Work out the finished part from the listing and answer in its coordinate system (mm). Face numbers are marked on the shaded views. Round coordinates to 2 decimals unless told otherwise and drop trailing zeros. Order: outer loops, then holes, each group sorted by start corner. A loop starts at its lowest first (then second) coordinate and runs counter-clockwise, first axis right, second up. Notation, with made-up numbers: (11.5, 76) - (68.5, 76) arc R35 cw to (68.5, 110) - close; hole circle Ø2 at (45.25, -7.75). An arc over 180 degrees is marked (long way). Answer in a Markdown table with one row per item.
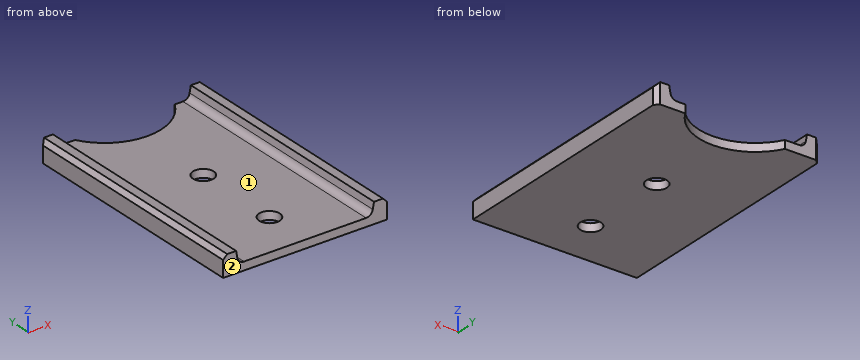
from build123d import *

# Parameters (mm, degrees)
F1_DEPTH = 228.6
F2_SIZE  = 3.81
F4_DEPTH = 25.4
F5_R     = 9.652
F6_DEPTH = 25.4


# Not quite as in the source:
# - a feature names something its author has since deleted; it is built from what else it names


with BuildPart() as f1:
    # F0 (on Front) → F1 (new body)
    with BuildSketch(Plane.XZ):
        with BuildLine():
            Line((-168.0421057219, 19.05), (-168.0421057219, 0))
            Line((-168.0421057219, 0), (-14.8801057219, 0))
            Line((-14.8801057219, 0), (-14.8801057219, 19.05))
            Line((-14.8801057219, 19.05), (-27.0467057219, 19.05))
            Line((-27.0467057219, 19.05), (-28.1368765378, 12.8673340718))
            ThreePointArc((-28.1368765378, 12.8673340718), (-30.3108938413, 9.1037793136), (-34.3961226724, 7.62))
            Line((-34.3961226724, 7.62), (-91.4611057219, 7.62))
            Line((-91.4611057219, 7.62), (-148.5260887714, 7.62))
            ThreePointArc((-148.5260887714, 7.62), (-152.6077900929, 9.1056177862), (-154.7796180031, 12.8673340718))
            Line((-154.7796180031, 12.8673340718), (-155.8697888189, 19.05))
            Line((-155.8697888189, 19.05), (-168.0421057219, 19.05))
        make_face()
    extrude(amount=F1_DEPTH)

    # F2
    f2_edges = [f1.edges().sort_by_distance(p)[0] for p in [
        (-168.042106, -114.3, 19.05),
        (-14.880106, -114.3, 19.05),
        (-14.880106, 0, 9.525),
        (-168.042106, 0, 9.525),
    ]]
    chamfer(f2_edges, length=F2_SIZE)

    # F3 (on face) → F4 (cut)
    with BuildSketch(Plane.XY.offset(7.62)):
        with BuildLine():
            Line((-42.1433808409, 0), (-135.2288363374, 0))
            ThreePointArc((-135.2288363374, 0), (-88.6861085892, -27.6225), (-42.1433808409, 0))
        make_face()
    extrude(amount=-F4_DEPTH, mode=Mode.SUBTRACT)

    # F5 (on face) → F6 (cut)
    with BuildSketch(Plane(origin=(0, 0, 0), x_dir=(1, 0, 0), z_dir=(0, 0, -1))):
        with Locations((-91.4611057219, 101.6)):
            Circle(F5_R)
        with Locations((-91.4611057219, 184.15)):
            Circle(F5_R)
    extrude(amount=-F6_DEPTH, mode=Mode.SUBTRACT)


solid = f1.part
1) Find the intervals of material crossed by probe 1 along X at (y, z) = (-101.6, 3.75); probe 2 along Y at (x, z) = (-94, 2.25); probe 3 along Z at (x, y) = (-103, -175), in increasing order. Write a range as from..to.
Filled in:
| item | result |
|---|---|
| probe 1 | x = -168.04..-101.11, -81.81..-14.88 |
| probe 2 | y = -228.6..-193.46, -174.84..-110.91, -92.29..-27.36 |
| probe 3 | z = 0..7.62 |
2) Find section D-D, the plane x = -139. Give the vertices of the cut face in (y, z).
Filled in:
| item | result |
|---|---|
| outline | (-228.6, 0) - (0, 0) - (0, 7.62) - (-228.6, 7.62) - close |
3) Each of these flat-tipped pins is pushed along its axis until it touches: pin 1 (12 mm diameter, centred on x = -72.5, y = -185, fed in from +Z); pin 2 (25 mm diameter, centred on x = -91.46, y = -184.15, fed in from -Z); pin 3 (12 mm diameter, centred on x = -146.5, y = -144, fed in from +Z); pin 4 (6 mm diameter, centred on x = -86, z = 8, fed in from +Y). Where does it stop, or does it pass through?
Filled in:
| item | result |
|---|---|
| pin 1 | stops at z = 7.62 |
| pin 2 | stops at z = 0 |
| pin 3 | stops at z = 9.02 |
| pin 4 | stops at y = -27.32 |
4) Find section C-C, the plane y = -73.5. Give the vertices of the cut face in (x, z).
Filled in:
| item | result |
|---|---|
| outline | (-168.04, 0) - (-14.88, 0) - (-14.88, 15.24) - (-18.69, 19.05) - (-27.05, 19.05) - (-28.14, 12.87) arc R6.35 cw to (-34.4, 7.62) - (-148.53, 7.62) arc R6.35 cw to (-154.78, 12.87) - (-155.87, 19.05) - (-164.23, 19.05) - (-168.04, 15.24) - close |
5) The mould has two halves that part along X. Classify the marked faces 1 and 2: released by +X, released by -X, zero draft, split by the parting line, or undercut.
Filled in:
| item | result |
|---|---|
| face 1 | undercut |
| face 2 | zero draft |
6) Find section B-B, the plane x = -88. Give the vertices of the cut face in (y, z).
Filled in:
| item | result |
|---|---|
| outline | (-228.6, 0) - (-193.16, 0) - (-193.16, 7.62) - (-228.6, 7.62) - close; (-175.14, 0) - (-110.61, 0) - (-110.61, 7.62) - (-175.14, 7.62) - close; (-92.59, 0) - (-27.62, 0) - (-27.62, 7.62) - (-92.59, 7.62) - close |
7) Find section A-A, the plane y = -184.15. Give the vertices of the cut face in (x, z), then the cut area to 3 significant figures.
Filled in:
| item | result |
|---|---|
| outline | (-168.04, 0) - (-101.11, 0) - (-101.11, 7.62) - (-148.53, 7.62) arc R6.35 cw to (-154.78, 12.87) - (-155.87, 19.05) - (-164.23, 19.05) - (-168.04, 15.24) - close; (-81.81, 0) - (-14.88, 0) - (-14.88, 15.24) - (-18.69, 19.05) - (-27.05, 19.05) - (-28.14, 12.87) arc R6.35 cw to (-34.4, 7.62) - (-81.81, 7.62) - close |
| area | 1,320 mm^2 |
